Design review of the part built by this model. Coordinates are the model's own, in mm. A direction names the side the tool comes from. Round coordinates to 2 decimals unless told otherwise and drop trailing zeros. Loops run counter-clockwise (first coordinate to the right, second up) from the corner with the lowest first, then second, coordinate; pieces in that order, holes last. Notation, with made-up numbers: (-6.5, 3) - (38.5, 3) arc R23 cw to (38.5, 30) - close; hole circle Ø3 at (77.5, -6.5). An arc over 180 degrees is marked (long way). Return JSON: item names as keys, results as strings. Group by question number.
from build123d import *

# Parameters (mm, degrees)
F0_W     = 20
F0_H     = 20
F0_R     = 8.25
F1_DEPTH = 24
F2_R     = 5
F3_R     = 4
F4_DEPTH = 6
F5_R     = 4
F6_DEPTH = 6


with BuildPart() as f1:
    # F0 (on Top) → F1 (new body)
    with BuildSketch(Plane.XY):
        Rectangle(F0_W, F0_H)
        Circle(F0_R, mode=Mode.SUBTRACT)
    extrude(amount=F1_DEPTH)

    # F2
    f2_edges = [f1.edges().sort_by_distance(p)[0] for p in [
        (10, 10, 12),
        (10, -10, 12),
        (-10, 10, 12),
        (-10, -10, 12),
    ]]
    fillet(f2_edges, radius=F2_R)

    # F3 (on face) → F4 (join)
    with BuildSketch(Plane.YZ.offset(10)):
        with Locations((0, 12)):
            Circle(F3_R)
    extrude(amount=F4_DEPTH)

    # F5 (on face) → F6 (join)
    with BuildSketch(Plane(origin=(-10, 0, 0), x_dir=(0, -1, 0), z_dir=(-1, 0, 0))):
        with Locations((0, 12)):
            Circle(F5_R)
    extrude(amount=F6_DEPTH)


solid = f1.part
Q1. Add section D-D, the plane y = -3. State the section outline as (x, z) points.
Q2. Add section C-C, the plane y = 0. State the section outline as (x, z) points.
Q3. Draft analysis for pull direction X (two halves, no side actions). For faces 4 (the cylindrical face through (8, -9, 12)), 5 (the flat face through (0, -10, 12)), 6 (the flat face through (-16, 0, 12)), 7 (the cylindrical face through (7.62, -3.16, 11.83)), state which applies: pulls with the +X half, pulls with the -X half, needs draft (parallel to the pull), parting line crosses it, or undercut.
Q4. For line 1 (Y direction, x = 0, z = 7); line 2 (Y direction, x = -4.5, z = 15), list the stretches that pass through material, from the lowest coordinate up.
Q5. Insertion check: pin 1 Ø4 at (y, z) = (-2.5, 3.5) entering from +X; pin 2 Ø12 at (x, z) = (-8, 9.5) entering from +Y; pin 3 Ø8 at (x, z) = (9.5, 12) entering from -Y. Each pin has a flat end and moves straight along its axis. Give the tip position at first contact, or say it passes through.
Q6. Add section B-B, the plane x = 0. State the section outline as (y, z) points, plus the area to 3 significant figures.
Q7. Add section A-A, the plane z = 12. State the section outline as (x, y) points, plus the area to 3 significant figures.
Q8. Tool access review of faces 1 (the cylindrical face through (-12.958, 0.521, 15.966)), 2 (the cylindrical face through (-9, 8, 12)), 3 (the cylindrical face through (12.958, -0.521, 15.966)): name each direction out of +Z, -Z, +X, -X, +Y, -Y from which nothing blocks a thin tool from reaching the whole face with its end or side.
Evaluation:
{
 "1": {"outline": "(-16, 9.35) - (-10, 9.35) - (-10, 0) - (-7.69, 0) - (-7.69, 24) - (-10, 24) - (-10, 14.65) - (-16, 14.65) - close; (7.69, 0) - (10, 0) - (10, 9.35) - (16, 9.35) - (16, 14.65) - (10, 14.65) - (10, 24) - (7.69, 24) - close"},
 "2": {"outline": "(-16, 8) - (-10, 8) - (-10, 0) - (-8.25, 0) - (-8.25, 24) - (-10, 24) - (-10, 16) - (-16, 16) - close; (8.25, 0) - (10, 0) - (10, 8) - (16, 8) - (16, 16) - (10, 16) - (10, 24) - (8.25, 24) - close"},
 "3": {"face 4": "pulls with the +X half", "face 5": "needs draft", "face 6": "pulls with the -X half", "face 7": "undercut"},
 "4": {"line 1": "-10 to -8.25, 8.25 to 10", "line 2": "-10 to -6.91, 6.91 to 10"},
 "5": {"pin 1": "x = 10", "pin 2": "y = 10", "pin 3": "y = -9.97"},
 "6": {"outline": "(-10, 0) - (-8.25, 0) - (-8.25, 24) - (-10, 24) - close; (8.25, 0) - (10, 0) - (10, 24) - (8.25, 24) - close", "area": "84.0 mm²"},
 "7": {"outline": "(-16, -4) - (-10, -4) - (-10, -5) arc R5 ccw to (-5, -10) - (5, -10) arc R5 ccw to (10, -5) - (10, -4) - (16, -4) - (16, 4) - (10, 4) - (10, 5) arc R5 ccw to (5, 10) - (-5, 10) arc R5 ccw to (-10, 5) - (-10, 4) - (-16, 4) - close; hole circle Ø16.5 at (0, 0)", "area": "261 mm²"},
 "8": {"face 1": "-X", "face 2": "+Z, -Z, -X, +Y", "face 3": "+X"}
}
